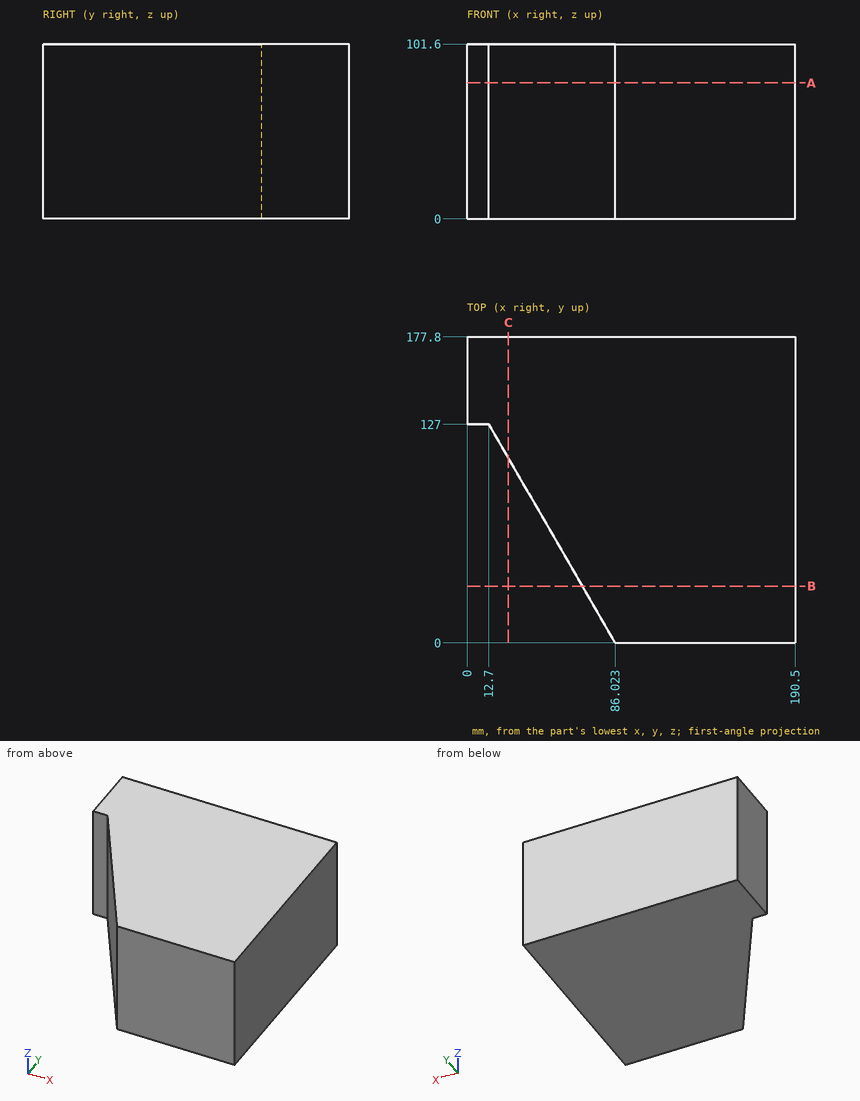
Input: dimensioned drawing with shaded views. Units: mm. Origin: part minimum x, y, z. Give positions to 0.01 mm unless a question says otherwise; leave off trailing zeros. Loops run counter-clockwise (first coordinate to the right, second up) from the corner with the lowest first, then second, coordinate; pieces in that order, holes last. Notation, with made-up numbers: M 31.5,-6.75 L 83.5,-6.75 A21 cw 83.5,-2.75 Z; hole C 66,-1.5 d8. An arc over 180 degrees is marked long. Put each result on its own line as item: value. Start each with the question number.
1) Cut plane A-A (z = 79). Output: boundary loops of the cut face in (x, y), then the cut area to 3 significant figures.
2) Cut plane B-B (y = 33). Output: boundary loops of the cut face in (x, z).
3) Contact query for flat-ended pins moving along their axis: pin 1 (2 mm diameter, centred on y = 63, z = 44, fed in from -X); pin 2 (5 mm diameter, centred on y = 34.5, z = 58, fed in from -X); pin 3 (10 mm diameter, centred on x = 6, z = 45, fed in from -Y). Output: stop coordinate, or through.
4) Cut plane C-C (x = 24). Output: boundary loops of the cut face in (y, z), then the cut area to 3 significant figures.
5) Ray query, line 1 along Y through (x, z) = (9, 48); line 2 along X through (y, z) = (109, 73.5); line 3 along X through (y, z) = (100, 62.5). Return the intervals inside material, ascending.
Verdict:
1. outline: M 0,127 L 12.7,127 L 86.02,0 L 190.5,0 L 190.5,177.8 L 0,177.8 Z
1. area: 27,600 mm2
2. outline: M 66.97,0 L 190.5,0 L 190.5,101.6 L 66.97,101.6 Z
3. pin 1: x = 49.07
3. pin 2: x = 64.66
3. pin 3: y = 127
4. outline: M 107.43,0 L 177.8,0 L 177.8,101.6 L 107.43,101.6 Z
4. area: 7,150 mm2
5. line 1: 127 to 177.8
5. line 2: 23.09 to 190.5
5. line 3: 28.29 to 190.5
